from build123d import *

# Parameters (mm, degrees)
F1_DEPTH = 57.15
F2_R     = 22.225
F3_DEPTH = 127
F4_R     = 11.43
F5_DEPTH = 76.2


with BuildPart() as f1:
    # F0 (on Top) → F1 (new body)
    with BuildSketch(Plane.XY):
        Polygon((0, 101.6), (0, 0), (127, 0), (127, 101.6), (101.6, 101.6), (101.6, 76.2), (25.4, 76.2), (25.4, 101.6), align=None)
    extrude(amount=F1_DEPTH)

    # F2 (on face) → F3 (cut)
    with BuildSketch(Plane.YZ.offset(127)):
        with Locations((101.6, 28.575)):
            Circle(F2_R)
    extrude(amount=-F3_DEPTH, mode=Mode.SUBTRACT)

    # F4 (on face) → F5 (cut)
    with BuildSketch(Plane.XY.offset(57.15)):
        with Locations((69.85, 38.1)):
            Circle(F4_R)
    extrude(amount=-F5_DEPTH, mode=Mode.SUBTRACT)


solid = f1.part
Check sheet for the modelled part. Datum: model origin and axes. Units: mm. A direction names the side the tool comes from. Give positions to 0.01 mm unless a question says otherwise; leave off trailing zeros. Order: outer loops, then holes, each group sorted by start corner. A loop starts at its lowest first (then second) coordinate and runs counter-clockwise, first axis right, second up. Notation, with made-up numbers: (30, 30.25) - (39, 30.25) arc R30 cw to (39, 64.25) - close; hole circle Ø11 at (65.5, -4). An arc over 180 degrees is marked (long way). Answer as CSV lines item,"result".
1. Section check A-A (y = 38.1). Record the boundary of the cut face in (x, z), then the cut area to 3 significant figures.
Result sheet:
outline,"(0, 0) - (58.42, 0) - (58.42, 57.15) - (0, 57.15) - close; (81.28, 0) - (127, 0) - (127, 57.15) - (81.28, 57.15) - close"
area,"5,950 mm²"
2. Section check B-B (x = 69.85). Record the boundary of the cut face in (y, z).
Result sheet:
outline,"(0, 0) - (26.67, 0) - (26.67, 57.15) - (0, 57.15) - close; (49.53, 0) - (76.2, 0) - (76.2, 57.15) - (49.53, 57.15) - close"
3. Section check D-D (x = 111). Record the boundary of the cut face in (y, z) (3 decimals), then the cut area to 3 significant figures.
Result sheet:
outline,"(0, 0) - (101.6, 0) - (101.6, 6.35) arc R22.225 cw to (101.6, 50.8) - (101.6, 57.15) - (0, 57.15) - close"
area,"5,030 mm²"
4. Go/stop test with a flat-tipped pin: P1, Ø17, axis at x = 49.5, z = 25, coming from the +Y side. Record where the tip stops, or that it passes through.
Result sheet:
P1,"y = 76.2"
5. Tool access check on faces 1 (the face through (13, 101.6, 3)), 2 (the face through (25.4, 77, 28)). Record the directions out of +Z, -Z, +X, -X, +Y, -Y that give a thin tool (end or side, any length) a straight path to the whole face; none if there is none.
Result sheet:
face 1,"+Z, -Z, +X, -X, +Y"
face 2,"+Z, -Z, +Y"
6. Section check C-C (z = 36). Record the boundary of the cut face in (x, y), then the cut area to 3 significant figures.
Result sheet:
outline,"(0, 0) - (127, 0) - (127, 80.65) - (101.6, 80.65) - (101.6, 76.2) - (25.4, 76.2) - (25.4, 80.65) - (0, 80.65) - close; hole circle Ø22.86 at (69.85, 38.1)"
area,"9,490 mm²"
7. Mould release check, pull along X, two halves, no side actions. Record for faces 3 (the face through (101.6, 78, 28)), 4 (the face through (63, 52, 0)), 5 (the face through (0, 40, 28)), 6 (the face through (127, 39, 28)): released by +X, released by -X, zero draft, split by the parting line, or undercut.
Result sheet:
face 3,"undercut"
face 4,"zero draft"
face 5,"released by -X"
face 6,"released by +X"
8. Scan lines: probe 1 along X at (y, z) = (38, 42); probe 2 along Y at (x, z) = (69, 21); probe 3 along Y at (x, z) = (36.5, 15.5). Record each from-to range of solid material in increasing order. Write a range as from..to.
Result sheet:
probe 1,"0..58.42, 81.28..127"
probe 2,"0..26.7, 49.5..76.2"
probe 3,"0..76.2"
